Verification items for the finished model (mm, model axes). Round coordinates to 2 decimals unless told otherwise and drop trailing zeros. Write each loop counter-clockwise with the first axis right and the second up, starting at its lowest first coordinate (ties: lowest second). Pieces come first, ordered by that corner, then holes. Notation, with made-up numbers: M 11.5,72 L 43.5,72 A12 ccw 43.5,89 Z; hole C -34.75,59.25 d9. An arc over 180 degrees is marked long. One line per item, written item: value. Start each with the question number.
Item 1: Section check B-B, the plane x = 78.5. Record the cut outline in (y, z).
Item 2: Gauge pin test, flat ends, axial feed: pin 1 (0.6 mm diameter, centred on x = 89.5, z = 1, fed in from -Y); pin 2 (1.5 mm diameter, centred on y = 44, z = 0.5, fed in from -X); pin 3 (1.1 mm diameter, centred on y = 24.5, z = 2.5, fed in from +X). Record the tip position at first contact, or that the pin passes through.
Item 3: Section check A-A, the plane x = 11.5. Record the cut outline in (y, z).
Item 4: Thickness scan on probe 1 along X at (y, z) = (31, 0.3); probe 2 along X at (y, z) = (27.5, 2.3); probe 3 along Y at (x, z) = (73.5, 1.1). Record the ranges inside material, lowest first. Write a range as from..to.
Item 5: Section check C-C, the plane z = 1.5. State how many separate pieces and enclosed holes the cut face has, then the cut area to 3 significant figures.
Item 6: Section check D-D, the plane x = 34. Record the cut outline in (y, z).
from build123d import *

# Parameters (mm, degrees)
SKETCH1_R            = 1.6
SKETCH1_R_2          = 2.1
BOSS_EXTRUDE3_DEPTH  = 2
BOSS_EXTRUDE4_DEPTH  = 2
SKETCH4_W            = 66
SKETCH4_H            = 16.340111315
SKETCH4_H_2          = 24.741581589
CUT_EXTRUDE3_DEPTH   = 14.5
FILLET1_R            = 4
SKETCH5_W            = 26
SKETCH5_H            = 27
SKETCH5_R            = 6
BOSS_EXTRUDE5_DEPTH  = 2
SKETCH6_W            = 5
SKETCH6_H            = 27
CUT_EXTRUDE4_DEPTH   = 14.5
SKETCH7_R            = 2.5
BOSS_EXTRUDE6_DEPTH  = 2
SKETCH8_R            = 2.5
CUT_EXTRUDE5_DEPTH   = 10
SKETCH9_W            = 22.081
SKETCH9_H            = 27
CUT_EXTRUDE6_DEPTH   = 10
CUT_EXTRUDE7_DEPTH   = 10
SKETCH11_W           = 28.061
SKETCH11_H           = 7.05
BOSS_EXTRUDE7_DEPTH  = 2
SKETCH12_W           = 44.061
SKETCH12_H           = 28.9
CUT_EXTRUDE9_DEPTH   = 10
BOSS_EXTRUDE9_DEPTH  = 2
FILLET2_R            = 4
SKETCH14_R           = 2.5
SKETCH14_W           = 28.061
SKETCH14_H           = 12.9
BOSS_EXTRUDE10_DEPTH = 1


with BuildPart() as part:
    # Sketch1 → Boss-Extrude3 (new body)
    with BuildSketch(Plane.XY):
        with BuildLine():
            Line((0, 3.5), (37.911912125, 3.5))
            Line((37.911912125, 3.5), (37.911912125, 13.97107578))
            Line((37.911912125, 13.97107578), (37.911912125, 40.97107578))
            Line((37.911912125, 40.97107578), (37.911912125, 51.44215156))
            Line((37.911912125, 51.44215156), (0, 51.44215156))
            ThreePointArc((0, 51.44215156), (-3.5, 54.94215156), (0, 58.44215156))
            Line((0, 58.44215156), (45.911912125, 58.44215156))
            Line((45.911912125, 58.44215156), (45.911912125, 51.44215156))
            Line((45.911912125, 51.44215156), (45.911912125, 48.97107578))
            Line((45.911912125, 48.97107578), (50.911912125, 48.97107578))
            Line((50.911912125, 48.97107578), (66.911912125, 48.97107578))
            Line((66.911912125, 48.97107578), (71.911912125, 48.97107578))
            Line((71.911912125, 48.97107578), (71.911912125, 51.44215156))
            Line((71.911912125, 51.44215156), (71.911912125, 58.44215156))
            Line((71.911912125, 58.44215156), (117.82382425, 58.44215156))
            ThreePointArc((117.82382425, 58.44215156), (121.32382425, 54.94215156), (117.82382425, 51.44215156))
            Line((117.82382425, 51.44215156), (79.911912125, 51.44215156))
            Line((79.911912125, 51.44215156), (79.911912125, 40.97107578))
            Line((79.911912125, 40.97107578), (79.911912125, 13.97107578))
            Line((79.911912125, 13.97107578), (79.911912125, 3.5))
            Line((79.911912125, 3.5), (117.82382425, 3.5))
            ThreePointArc((117.82382425, 3.5), (121.32382425, 0), (117.82382425, -3.5))
            Line((117.82382425, -3.5), (71.911912125, -3.5))
            Line((71.911912125, -3.5), (71.911912125, 3.5))
            Line((71.911912125, 3.5), (71.911912125, 5.97107578))
            Line((71.911912125, 5.97107578), (66.911912125, 5.97107578))
            Line((66.911912125, 5.97107578), (50.911912125, 5.97107578))
            Line((50.911912125, 5.97107578), (45.911912125, 5.97107578))
            Line((45.911912125, 5.97107578), (45.911912125, 3.5))
            Line((45.911912125, 3.5), (45.911912125, -3.5))
            Line((45.911912125, -3.5), (0, -3.5))
            ThreePointArc((0, -3.5), (-3.5, 0), (0, 3.5))
        make_face()
        with Locations((0, 54.94215156)):
            Circle(SKETCH1_R, mode=Mode.SUBTRACT)
        with Locations((117.82382425, 54.94215156)):
            Circle(SKETCH1_R, mode=Mode.SUBTRACT)
        with Locations((117.82382425, 0)):
            Circle(SKETCH1_R, mode=Mode.SUBTRACT)
        Circle(SKETCH1_R, mode=Mode.SUBTRACT)
        with Locations((66.911912125, 44.97107578)):
            Circle(SKETCH1_R_2, mode=Mode.SUBTRACT)
        with Locations((66.911912125, 9.97107578)):
            Circle(SKETCH1_R_2, mode=Mode.SUBTRACT)
        with Locations((50.911912125, 9.97107578)):
            Circle(SKETCH1_R_2, mode=Mode.SUBTRACT)
        with Locations((50.911912125, 44.97107578)):
            Circle(SKETCH1_R_2, mode=Mode.SUBTRACT)
        Polygon((66.911912125, 40.97107578), (50.911912125, 40.97107578), (45.911912125, 40.97107578), (45.911912125, 27.47107578), (45.911912125, 13.97107578), (50.911912125, 13.97107578), (66.911912125, 13.97107578), (71.911912125, 13.97107578), (71.911912125, 27.47107578), (71.911912125, 40.97107578), align=None, mode=Mode.SUBTRACT)
    extrude(amount=BOSS_EXTRUDE3_DEPTH)

    # Sketch3 → Boss-Extrude4 (add)
    with BuildSketch(Plane.XY.offset(2)):
        Polygon((71.911912125, 13.97107578), (99.911912125, 13.97107578), (99.911912125, 3.5), (91.911912125, 3.5), (91.911912125, 5.97107578), (71.911912125, 5.97107578), align=None)
        Polygon((91.911912125, 51.44215156), (99.911912125, 51.44215156), (99.911912125, 40.97107578), (71.911912125, 40.97107578), (71.911912125, 48.97107578), (91.911912125, 48.97107578), align=None)
        Polygon((45.911912125, 40.97107578), (17.911912125, 40.97107578), (17.911912125, 51.44215156), (25.911912125, 51.44215156), (25.911912125, 48.97107578), (45.911912125, 48.97107578), align=None)
        Polygon((25.911912125, 3.5), (17.911912125, 3.5), (17.911912125, 13.97107578), (45.911912125, 13.97107578), (45.911912125, 5.97107578), (25.911912125, 5.97107578), align=None)
    extrude(amount=-BOSS_EXTRUDE4_DEPTH)

    # Sketch4 → Cut-Extrude3 (cut)
    with BuildSketch(Plane.XY.offset(2)):
        with Locations((58.911912125, 57.141131438)):
            Rectangle(SKETCH4_W, SKETCH4_H)
        with Locations((58.911912125, -6.399715014)):
            Rectangle(SKETCH4_W, SKETCH4_H_2)
    extrude(amount=-CUT_EXTRUDE3_DEPTH, mode=Mode.SUBTRACT)

    # Fillet1
    fillet1_edges = [part.edges().sort_by_distance(p)[0] for p in [
        (99.911912125, 13.97107578, 1),
        (99.911912125, 3.5, 1),
        (91.911912125, 5.97107578, 1),
        (91.911912125, 48.97107578, 1),
        (99.911912125, 51.44215156, 1),
        (99.911912125, 40.97107578, 1),
        (17.911912125, 40.97107578, 1),
        (17.911912125, 51.44215156, 1),
        (25.911912125, 48.97107578, 1),
        (25.911912125, 5.97107578, 1),
        (17.911912125, 3.5, 1),
        (17.911912125, 13.97107578, 1),
        (91.911912125, 58.44215156, 1),
        (25.911912125, 58.44215156, 1),
        (91.911912125, -3.5, 1),
        (25.911912125, -3.5, 1),
    ]]
    fillet(fillet1_edges, radius=FILLET1_R)

    # Sketch5 → Boss-Extrude5 (add)
    with BuildSketch(Plane.XY.offset(2)):
        with Locations((58.911912125, 27.47107578)):
            Rectangle(SKETCH5_W, SKETCH5_H)
        with Locations((58.911912125, 27.47107578)):
            Circle(SKETCH5_R, mode=Mode.SUBTRACT)
    extrude(amount=-BOSS_EXTRUDE5_DEPTH)

    # Sketch6 → Cut-Extrude4 (cut)
    with BuildSketch(Plane.XY.offset(2)):
        with Locations((40.411912125, 27.47107578)):
            Rectangle(SKETCH6_W, SKETCH6_H)
        with Locations((77.411912125, 27.47107578)):
            Rectangle(SKETCH6_W, SKETCH6_H)
    extrude(amount=-CUT_EXTRUDE4_DEPTH, mode=Mode.SUBTRACT)

    # Sketch7 → Boss-Extrude6 (add)
    with BuildSketch(Plane.XY.offset(2)):
        Polygon((80.891912125, 27.47107578), (80.891912125, 40.97107578), (88.891912125, 40.97107578), (88.891912125, 27.47107578), (88.891912125, 13.97107578), (80.891912125, 13.97107578), align=None)
        with Locations((84.891912125, 27.47107578)):
            Circle(SKETCH7_R, mode=Mode.SUBTRACT)
    extrude(amount=-BOSS_EXTRUDE6_DEPTH)

    # Sketch8 → Cut-Extrude5 (cut)
    with BuildSketch(Plane.XY.offset(2)):
        with Locations((48.830912125, 27.47107578)):
            Circle(SKETCH8_R)
    extrude(amount=-CUT_EXTRUDE5_DEPTH, mode=Mode.SUBTRACT)

    # Sketch9 → Cut-Extrude6 (cut)
    with BuildSketch(Plane.XY.offset(2)):
        Polygon((42.911912125, 40.97107578), (44.830912125, 40.97107578), (44.830912125, 27.47107578), (44.830912125, 13.97107578), (42.911912125, 13.97107578), align=None)
        with Locations((63.871412125, 27.47107578)):
            Rectangle(SKETCH9_W, SKETCH9_H)
    extrude(amount=-CUT_EXTRUDE6_DEPTH, mode=Mode.SUBTRACT)

    # Sketch10 → Cut-Extrude7 (cut)
    with BuildSketch(Plane.XY.offset(2)):
        Polygon((44.830912125, 13.97107578), (44.830912125, 13.02107578), (88.891912125, 13.02107578), (88.891912125, 13.97107578), (106.020559472, 13.97107578), (106.020559472, 3.5), (12.964535502, 3.5), (12.964535502, 13.97107578), align=None)
        Polygon((88.891912125, 40.97107578), (88.891912125, 41.92107578), (44.830912125, 41.92107578), (44.830912125, 40.97107578), (12.964535502, 40.97107578), (12.964535502, 51.44215156), (106.020559472, 51.44215156), (106.020559472, 40.97107578), align=None)
    extrude(amount=-CUT_EXTRUDE7_DEPTH, mode=Mode.SUBTRACT)

    # Sketch11 → Boss-Extrude7 (add)
    with BuildSketch(Plane.XY.offset(2)):
        with Locations((66.861412125, 37.44607578)):
            Rectangle(SKETCH11_W, SKETCH11_H)
        with Locations((66.861412125, 17.49607578)):
            Rectangle(SKETCH11_W, SKETCH11_H)
    extrude(amount=-BOSS_EXTRUDE7_DEPTH)

    # Sketch12 → Cut-Extrude9 (cut)
    with BuildSketch(Plane.XY.offset(2)):
        Polygon((25.911912125, 1.23553789), (25.911912125, 54.44215156), (91.911912125, 54.44215156), (91.911912125, 0.5), align=None)
        with Locations((66.861412125, 27.47107578)):
            Rectangle(SKETCH12_W, SKETCH12_H, mode=Mode.SUBTRACT)
    extrude(amount=-CUT_EXTRUDE9_DEPTH, mode=Mode.SUBTRACT)

    # Sketch13 → Boss-Extrude9 (add)
    with BuildSketch(Plane.XY.offset(2)):
        Polygon((17.911912125, 3.5), (25.911912125, 3.5), (25.911912125, 13.02107578), (44.830912125, 13.02107578), (44.830912125, 21.02107578), (25.911912125, 21.02107578), (25.911912125, 33.92107578), (44.830912125, 33.92107578), (44.830912125, 41.92107578), (25.911912125, 41.92107578), (25.911912125, 51.44215156), (17.911912125, 51.44215156), (17.911912125, 13.02107578), align=None)
        Polygon((99.911912125, 51.44215156), (91.911912125, 51.44215156), (91.911912125, 41.92107578), (88.891912125, 41.92107578), (88.891912125, 33.92107578), (91.911912125, 33.92107578), (91.911912125, 21.02107578), (88.891912125, 21.02107578), (88.891912125, 13.02107578), (91.911912125, 13.02107578), (91.911912125, 3.5), (99.911912125, 3.5), (99.911912125, 41.92107578), align=None)
    extrude(amount=-BOSS_EXTRUDE9_DEPTH)

    # Fillet2
    fillet2_edges = [part.edges().sort_by_distance(p)[0] for p in [
        (99.911912125, 51.44215156, 1),
        (99.911912125, 3.5, 1),
        (91.911912125, 13.02107578, 1),
        (91.911912125, 41.92107578, 1),
        (25.911912125, 13.02107578, 1),
        (17.911912125, 3.5, 1),
        (17.911912125, 51.44215156, 1),
        (25.911912125, 41.92107578, 1),
    ]]
    fillet(fillet2_edges, radius=FILLET2_R)

    # Sketch14 → Boss-Extrude10 (add)
    with BuildSketch(Plane.XY.offset(2)):
        Polygon((44.830912125, 33.92107578), (44.830912125, 37.92107578), (88.891912125, 37.92107578), (88.891912125, 33.92107578), (88.891912125, 21.02107578), (88.891912125, 16.479152283), (44.830912125, 16.479152283), (44.830912125, 21.02107578), align=None)
        with Locations((48.830912125, 27.47107578)):
            Circle(SKETCH14_R, mode=Mode.SUBTRACT)
        with Locations((84.891912125, 27.47107578)):
            Circle(SKETCH14_R, mode=Mode.SUBTRACT)
        with Locations((66.861412125, 27.47107578)):
            Rectangle(SKETCH14_W, SKETCH14_H, mode=Mode.SUBTRACT)
    extrude(amount=BOSS_EXTRUDE10_DEPTH)


solid = part.part
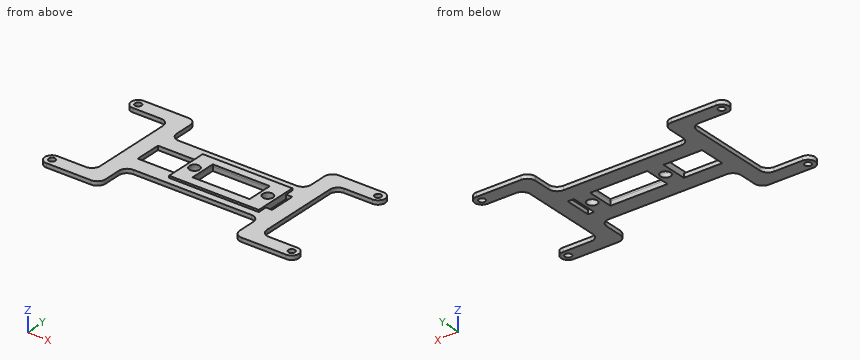
Response values:
1. outline: M 13.02,0 L 21.02,0 L 21.02,3 L 16.48,3 L 16.48,2 L 13.02,2 Z; M 33.92,0 L 41.92,0 L 41.92,2 L 37.92,2 L 37.92,3 L 33.92,3 Z
2. pin 1: stops at y = 12.55
2. pin 2: stops at x = 17.91
2. pin 3: stops at x = 99.91
3. outline: M -3.5,0 L 3.5,0 L 3.5,2 L -3.5,2 Z; M 51.44,0 L 58.44,0 L 58.44,2 L 51.44,2 Z
4. probe 1: x = 17.91..25.91, 44.83..52.83, 80.89..88.89, 91.91..99.91
4. probe 2: x = 44.83..46.33, 51.33..52.83, 80.89..82.39, 87.39..88.89
4. probe 3: y = 13.02..21.02, 33.92..41.92
5. separate pieces: 1
5. enclosed holes: 9
5. area: 2,770 mm2
6. outline: M 13.02,0 L 21.02,0 L 21.02,2 L 13.02,2 Z; M 33.92,0 L 41.92,0 L 41.92,2 L 33.92,2 Z
